Answer from the drawing. Dimensions are ordinates in mm from the lowest x, y and z of the part. A direction names the side the tool comes from. Round coordinates to 2 decimals unless told otherwise and drop trailing zeros. Write each loop counter-clockwise with the first axis right and the second up, starting at its lowest first coordinate (ties: lowest second). Pieces come first, ordered by that corner, then holes. Notation, with made-up numbers: (-40, -36.5) - (14, -36.5) arc R18 ccw to (14, -18.5) - close; hole circle Ø5 at (38, 49). An arc over 180 degrees is marked (long way). Answer in a Markdown table with one row per item.
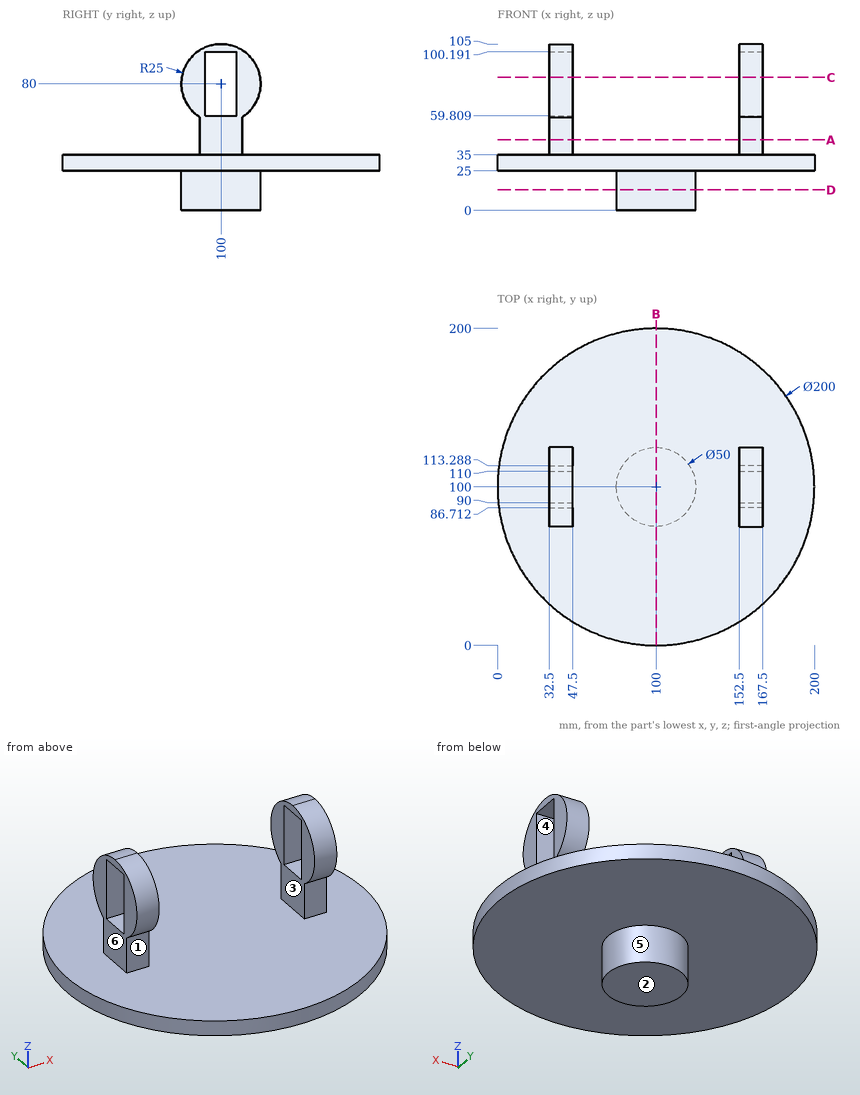
(1) Flat-ended cylindrical pins translate along their axes: pin 1 (5 mm diameter, centred on x = 53, z = 27, fed in from +Y); pin 2 (1 mm diameter, centred on y = 110.5, z = 91, fed in from -X); pin 3 (12 mm diameter, centred on x = 159.5, z = 47.5, fed in from -Y). Find the tip coordinate at first contact, or state that the pin passes through.
Checked values:
| item | result |
|---|---|
| pin 1 | stops at y = 189.55 |
| pin 2 | stops at x = 32.5 |
| pin 3 | stops at y = 86.71 |
(2) Section A-A (z = 44.5) is taken. Give the vertices of the cut face in (x, y), and give its area (3 significant figures).
Checked values:
| item | result |
|---|---|
| outline | (32.5, 86.71) - (47.5, 86.71) - (47.5, 113.29) - (32.5, 113.29) - close; (152.5, 86.71) - (167.5, 86.71) - (167.5, 113.29) - (152.5, 113.29) - close |
| area | 797 mm2 |
(3) Find the intervals of material crossed by line 1 (X direction, y = 92, z = 59.5); line 2 (Z direction, x = 77.5, y = 13); line 3 (Y direction, x = 47, z = 79.5) (3 decimals), in increasing order.
Checked values:
| item | result |
|---|---|
| line 1 | x = 32.5 to 47.5, 152.5 to 167.5 |
| line 2 | z = 25 to 35 |
| line 3 | y = 75.005 to 90, 110 to 124.995 |
(4) Section B-B (x = 100) is taken. Give the vertices of the cut face in (y, z).
Checked values:
| item | result |
|---|---|
| outline | (0, 25) - (75, 25) - (75, 0) - (125, 0) - (125, 25) - (200, 25) - (200, 35) - (0, 35) - close |
(5) Section D-D (z = 13) is taken. Give the vertices of the cut face in (x, y), and give its area (3 significant figures).
Checked values:
| item | result |
|---|---|
| outline | circle Ø50 at (100, 100) |
| area | 1,960 mm2 |
(6) For a pull along Z with two mould halves and no side action, classify the marked faces 1, 2 and 3 as pulls with the +Z half, pulls with the -Z half, needs draft (parallel to the pull), parting line crosses it, or undercut.
Checked values:
| item | result |
|---|---|
| face 1 | undercut |
| face 2 | pulls with the -Z half |
| face 3 | needs draft |
(7) For the marked faces 4, 5 and 6, determine the directions among +Z, -Z, +X, -X, +Y, -Y from which every point of the face is accessible in a straight line to the end or side of a thin tool.
Checked values:
| item | result |
|---|---|
| face 4 | +X, -X |
| face 5 | -Z |
| face 6 | +Z, -X, +Y, -Y |
(8) Section C-C (z = 84) is taken. Give the vertices of the cut face in (x, y), and give its area (3 significant figures).
Checked values:
| item | result |
|---|---|
| outline | (32.5, 75.32) - (47.5, 75.32) - (47.5, 90) - (32.5, 90) - close; (32.5, 110) - (47.5, 110) - (47.5, 124.68) - (32.5, 124.68) - close; (152.5, 75.32) - (167.5, 75.32) - (167.5, 90) - (152.5, 90) - close; (152.5, 110) - (167.5, 110) - (167.5, 124.68) - (152.5, 124.68) - close |
| area | 881 mm2 |
